Can you work these out from the model? Positions are in its coordinate system, mm. A direction names the side the tool comes from. Give positions to 0.01 mm unless a question says otherwise; leave off trailing zeros. Loops run counter-clockwise (first coordinate to the right, second up) from the corner with the lowest first, then second, coordinate; pieces in that order, holes last. Notation, with made-up numbers: M 86,34.25 L 111,34.25 A23 ccw 111,65.25 Z; hole C 20,-21.5 d9. An arc over 180 degrees is marked long. Use CSV: the item, a comma, the result in double quotes.
from build123d import *

# Parameters (mm, degrees)
ESBO_O1_W                   = 100
ESBO_O1_H                   = 100
RESSALTO_EXTRUS_O1_DEPTH    = 20
CORTE_EXTRUS_O1_DEPTH       = 74.484692283
CORTE_EXTRUS_O1_DEPTH_BACK  = 74.484692283
ESBO_O2_R                   = 20
ESBO_O3_W                   = 94
ESBO_O3_H                   = 74
CORTE_EXTRUS_O2_DEPTH       = 74.484692283
ESBO_O5_W                   = 94
ESBO_O5_H                   = 74
CORTE_EXTRUS_O3_DEPTH       = 17
CORTE_EXTRUS_O4_START       = 50
ESBO_O6_R                   = 16
CORTE_EXTRUS_O4_DEPTH       = 21
CORTE_EXTRUS_O5_START       = -29
ESBO_O6_4_R                 = 16
CORTE_EXTRUS_O5_DEPTH       = 21
ESBO_O7_W                   = 21
ESBO_O7_H                   = 3.872983347
CORTE_EXTRUS_O6_DEPTH       = 21
ESBO_O8_R                   = 1.5
ESBO_O8_W                   = 4.5
ESBO_O8_H                   = 2.5
CORTE_EXTRUS_O8_DEPTH       = 74.484692283
ESBO_O9_R                   = 1.5
ESBO_O9_W                   = 4.5
ESBO_O9_H                   = 2.5
CORTE_EXTRUS_O9_DEPTH       = 74.484692283
CORTE_EXTRUS_O10_DEPTH      = 74.484692283
CORTE_EXTRUS_O10_DEPTH_BACK = 74.484692283
ESBO_O10_R                  = 1.5
ESBO_O10_W                  = 4.5
ESBO_O10_H                  = 2.5


with BuildPart() as part:
    # Esboço1 → Ressalto-extrusão1 (new, symmetric)
    with BuildSketch(Plane(origin=(0, 0, 0), x_dir=(1, 0, 0), z_dir=(0, 1, 0))):
        Rectangle(ESBO_O1_W, ESBO_O1_H)
    extrude(amount=RESSALTO_EXTRUS_O1_DEPTH, both=True)

    # Esboço2 → Corte-extrusão1 (cut, two sides: drawn at the far end of the back side and taken through both)
    with BuildSketch(Plane(origin=(0, 0, 0), x_dir=(0, 0, -1), z_dir=(1, 0, 0)).offset(-CORTE_EXTRUS_O1_DEPTH_BACK)):
        with BuildLine():
            Line((-30, 20), (-50, 20))
            ThreePointArc((-50, 20), (-35.857864376, 14.142135624), (-30, 0))
            Line((-30, 0), (-30, 20))
        make_face()
        with Locations((-50, 0)):
            Circle(ESBO_O2_R)
    extrude(amount=CORTE_EXTRUS_O1_DEPTH + CORTE_EXTRUS_O1_DEPTH_BACK, mode=Mode.SUBTRACT)

    # Esboço3 → Corte-extrusão2 (cut, through all)
    with BuildSketch(Plane(origin=(0, 0, 0), x_dir=(1, 0, 0), z_dir=(0, 1, 0))):
        with Locations((0, 10)):
            Rectangle(ESBO_O3_W, ESBO_O3_H)
    extrude(amount=CORTE_EXTRUS_O2_DEPTH, mode=Mode.SUBTRACT)

    # Esboço5 → Corte-extrusão3 (cut)
    with BuildSketch(Plane(origin=(0, 0, 0), x_dir=(1, 0, 0), z_dir=(0, 1, 0))):
        with Locations((0, 10)):
            Rectangle(ESBO_O5_W, ESBO_O5_H)
    extrude(amount=-CORTE_EXTRUS_O3_DEPTH, mode=Mode.SUBTRACT)

    # Esboço6 → Corte-extrusão4 (cut)
    with BuildSketch(Plane(origin=(0, 0, 0), x_dir=(0, 0, -1), z_dir=(1, 0, 0)).offset(CORTE_EXTRUS_O4_START)):
        with Locations((36, -6)):
            Circle(ESBO_O6_R)
        with BuildLine():
            ThreePointArc((52, -6), (47.313708499, -17.313708499), (36, -22))
            Line((36, -22), (52, -22))
            Line((52, -22), (52, -6))
        make_face()
    extrude(amount=-CORTE_EXTRUS_O4_DEPTH, mode=Mode.SUBTRACT)

    # Esboço6<4> → Corte-extrusão5 (cut)
    with BuildSketch(Plane(origin=(0, 0, 0), x_dir=(0, 0, -1), z_dir=(1, 0, 0)).offset(CORTE_EXTRUS_O5_START)):
        with BuildLine():
            ThreePointArc((52, -6), (47.313708499, -17.313708499), (36, -22))
            Line((36, -22), (52, -22))
            Line((52, -22), (52, -6))
        make_face()
        with Locations((36, -6)):
            Circle(ESBO_O6_4_R)
    extrude(amount=-CORTE_EXTRUS_O5_DEPTH, mode=Mode.SUBTRACT)

    # Esboço7 → Corte-extrusão6 (cut)
    with BuildSketch(Plane(origin=(0, 0, 0), x_dir=(1, 0, 0), z_dir=(0, 1, 0))):
        with Locations((-39.5, 26.317541635)):
            Rectangle(ESBO_O7_W, ESBO_O7_H)
        with Locations((39.5, 26.317541635)):
            Rectangle(ESBO_O7_W, ESBO_O7_H)
    extrude(amount=-CORTE_EXTRUS_O6_DEPTH, mode=Mode.SUBTRACT)

    # Esboço8 → Corte-extrusão8 (cut, through all)
    with BuildSketch(Plane.XY):
        with Locations(Location((-43, 10, 0), (0, 0, 180))):
            Circle(ESBO_O8_R)
        with Locations(Location((-23.5, 10, 0), (0, 0, 180))):
            Circle(ESBO_O8_R)
        with Locations(Location((23.5, 10, 0), (0, 0, 180))):
            Circle(ESBO_O8_R)
        with Locations(Location((43, 10, 0), (0, 0, 180))):
            Circle(ESBO_O8_R)
        with Locations((33.25, 12)):
            Rectangle(ESBO_O8_W, ESBO_O8_H)
        with Locations((-33.25, 12)):
            Rectangle(ESBO_O8_W, ESBO_O8_H)
    extrude(amount=CORTE_EXTRUS_O8_DEPTH, mode=Mode.SUBTRACT)

    # Esboço9 → Corte-extrusão9 (cut, through all)
    with BuildSketch(Plane.XY):
        with Locations((-9.75, 10)):
            Circle(ESBO_O9_R)
        with Locations((9.75, 10)):
            Circle(ESBO_O9_R)
        with Locations((0, 12)):
            Rectangle(ESBO_O9_W, ESBO_O9_H)
    extrude(amount=-CORTE_EXTRUS_O9_DEPTH, mode=Mode.SUBTRACT)

    # Esboço10 → Corte-extrusão10 (cut, two sides: drawn at the far end of the back side and taken through both)
    with BuildSketch(Plane(origin=(0, 0, 0), x_dir=(0, 0, -1), z_dir=(1, 0, 0)).offset(-CORTE_EXTRUS_O10_DEPTH_BACK)):
        with Locations((-12, 10)):
            Circle(ESBO_O10_R)
        with Locations((7.5, 10)):
            Circle(ESBO_O10_R)
        with Locations((-2.25, 12)):
            Rectangle(ESBO_O10_W, ESBO_O10_H)
    extrude(amount=CORTE_EXTRUS_O10_DEPTH + CORTE_EXTRUS_O10_DEPTH_BACK, mode=Mode.SUBTRACT)


solid = part.part
Q1. I want a section at B-B, the plane y = -2. Please give me the cut outline in (x, z), then the cut area to 3 significant figures.
Model answer:
outline,"M -50,-20.51 L -47,-20.51 L -47,27 L 47,27 L 47,-20.51 L 50,-20.51 L 50,30.1 L -50,30.1 Z; M -29,-50 L 29,-50 L 29,-47 L -29,-47 Z"
area,"769 mm2"
Q2. If we mould it in two halves opening along Z, with no side actions, what happens to faces 1 (the flat face through (48, 12, 4.5)), 2 (the flat face through (39, -18, -24.381)), 3 (the flat face through (-1, -20, -1))? For each: released by +Z, released by -Z, zero draft, split by the parting line, or undercut.
Model answer:
face 1,"undercut"
face 2,"released by -Z"
face 3,"zero draft"
Q3. I want a section at C-C, the plane x = -43. Please give me the cut outline in (y, z), then the cut area to 3 significant figures.
Model answer:
outline,"M -20,-24.38 L -17,-24.38 L -17,27 L 8.5,27 L 8.5,30 L 0,30 A20 cw -20,50 Z; M 1.75,-50 L 20,-50 L 20,-47 L 5.62,-47 A16 cw Z; M 11.5,27 L 20,27 L 20,30 L 11.5,30 Z"
area,"399 mm2"
Q4. For faces 4 (the flat face through (0, 10.75, -48)), 5 (the cylindrical face through (-47.229, 9.864, -38.082)), 6 (the flat face through (-49, 13.25, 2)), 7 (the flat face through (-33, 10.75, 28)), which set-ups out of +Z, -Z, +X, -X, +Y, -Y let a thin tool reach every point of the face, with its end or its side?
Model answer:
face 4,"-Z"
face 5,"-X"
face 6,"+X, -X"
face 7,"+Z"
Q5. I want a section at A-A, the plane x = 23.5. Please give me the cut outline in (y, z).
Model answer:
outline,"M -20,-50 L 20,-50 L 20,-47 L -17,-47 L -17,27 L 8.5,27 L 8.5,30 L 0,30 A20 cw -20,50 Z; M 11.5,27 L 20,27 L 20,30 L 11.5,30 Z"
Q6. I'm going to push flat-ended pins straight in: P1, Ø0.9, axis at x = 44.5, y = -19, coming from the -Z side; P2, Ø8, axis at x = -13.5, y = 2, coming from the +Z side; P3, Ø2.5, axis at x = 43, y = 10, coming from the +Z side; P4, Ø6, axis at y = -12.5, z = -37, coming from the +X side. Where does each tip first touch, or does it pass through?
Model answer:
P1,"z = -24.38"
P2,"z = 30.1"
P3,"z = -47"
P4,"through"
Q7. I want a section at D-D, the plane z = 24. Please give me the cut outline in (x, y).
Model answer:
outline,"M -50,-20 L 50,-20 L 50,20 L 47,20 L 47,-17 L -47,-17 L -47,20 L -50,20 Z"
Q8. Please list where these lines run through material, in increasing order: L1, parallel to X at y = 7, z = -12.5; L2, parallel to Y at x = -49, z = 12; L3, parallel to Z at x = 19.5, y = 18.5. Write a range as from..to.
Model answer:
L1,"-50..-47, 47..50"
L2,"-20..8.5, 11.5..20"
L3,"-50..-47, 27..30"
